Here's how the part is built. I have some questions about the finished solid (model axes, mm). A direction names the side the tool comes from. Round coordinates to 2 decimals unless told otherwise and drop trailing zeros. Loops run counter-clockwise (first coordinate to the right, second up) from the corner with the lowest first, then second, coordinate; pieces in that order, holes last. Notation, with made-up numbers: M 4.5,9 L 12.5,9 A7 ccw 12.5,17 Z; hole C 6,28.5 d5. An arc over 180 degrees is marked long. Answer as CSV lines item,"result".
```python
from build123d import *

# Parameters (mm, degrees)
PAD_DEPTH     = 22
SKETCH001_R   = 5
SKETCH001_R_2 = 2.5
PAD001_DEPTH  = 0.4


with BuildPart() as part:
    # Sketch → Pad (new body)
    with BuildSketch(Plane.XY):
        Polygon((4.041452, -7), (8.082904, 0), (4.041452, 7), (-4.041452, 7), (-8.082904, 0), (-4.041452, -7), align=None)
        Polygon((4.676537, 0), (2.338269, 4.05), (-2.338269, 4.05), (-4.676537, 0), (-2.338269, -4.05), (2.338269, -4.05), align=None, mode=Mode.SUBTRACT)
    extrude(amount=PAD_DEPTH)

    # Sketch001 → Pad001 (join)
    with BuildSketch(Plane.XY):
        Circle(SKETCH001_R)
        Circle(SKETCH001_R_2, mode=Mode.SUBTRACT)
    extrude(amount=PAD001_DEPTH)


solid = part.part
```
1. Which directions (+Z, -Z, +X, -X, +Y, -Y) give clear straight access to the entire face, cutting with the end or side of a thin tool? Please do faces 1 (the flat face through (-3.491, 2.053, 11.049)), 2 (the flat face through (6.09, 3.45, 10.85)).
Evaluation:
face 1,"+Z"
face 2,"+Z, -Z, +X, +Y"
2. For P1, Ø2.5, axis at x = -0.5, y = -2, coming from the +Z side; P2, Ø3, axis at x = -5, y = 4.5, coming from the -Z side; P3, Ø2, axis at y = 2, z = 9.5, coming from the -X side; P4, Ø6, axis at y = 2, z = 13, coming from the +X side, each with a flat end and sliding along its axis, tell me the tip position at first contact or that it passes through.
Evaluation:
P1,"stops at z = 0.4"
P2,"stops at z = 0"
P3,"stops at x = -7.51"
P4,"stops at x = 8.08"
3. If I drill on line 1 (Y direction, x = 0, z = 0.1); line 2 (Y direction, x = 1, z = 7.5); line 3 (X direction, y = 2, z = 10.75), over which ranges is the centre line in solid material (lowest first)? Write a range as [from, to].
Evaluation:
line 1,"y = [-7, -2.5], [2.5, 7]"
line 2,"y = [-7, -4.05], [4.05, 7]"
line 3,"x = [-6.93, -3.52], [3.52, 6.93]"
4. I want a section at C-C, the plane y = 2.25. Please give me the cut outline in (x, z), and give its area (3 significant figures).
Evaluation:
outline,"M -6.78,0 L -1.09,0 L -1.09,0.4 L -3.38,0.4 L -3.38,22 L -6.78,22 Z; M 1.09,0 L 6.78,0 L 6.78,22 L 3.38,22 L 3.38,0.4 L 1.09,0.4 Z"
area,"152 mm²"
5. I want a section at A-A, the plane z = 11.25. Please give me the cut outline in (x, y).
Evaluation:
outline,"M -8.08,0 L -4.04,-7 L 4.04,-7 L 8.08,0 L 4.04,7 L -4.04,7 Z; hole M -4.68,0 L -2.34,-4.05 L 2.34,-4.05 L 4.68,0 L 2.34,4.05 L -2.34,4.05 Z"
6. I want a section at B-B, the plane x = 0. Please give me the cut outline in (y, z).
Evaluation:
outline,"M -7,0 L -2.5,0 L -2.5,0.4 L -4.05,0.4 L -4.05,22 L -7,22 Z; M 2.5,0 L 7,0 L 7,22 L 4.05,22 L 4.05,0.4 L 2.5,0.4 Z"
7. I want a section at D-D, the plane y = -3.5. Please give me the cut outline in (x, z).
Evaluation:
outline,"M -6.06,0 L 6.06,0 L 6.06,22 L 2.66,22 L 2.66,0.4 L -2.66,0.4 L -2.66,22 L -6.06,22 Z"
8. We'd pull the mould along X, two halves only. Please class faces 3 (the flat face through (0, 7, 11)), 4 (the cylindrical face through (-0.54, -2.44, 0.2)), 5 (the flat face through (6.034, -3.549, 10.846)): pulls with the +X half, pulls with the -X half, needs draft (parallel to the pull), parting line crosses it, or undercut.
Evaluation:
face 3,"needs draft"
face 4,"undercut"
face 5,"pulls with the +X half"
